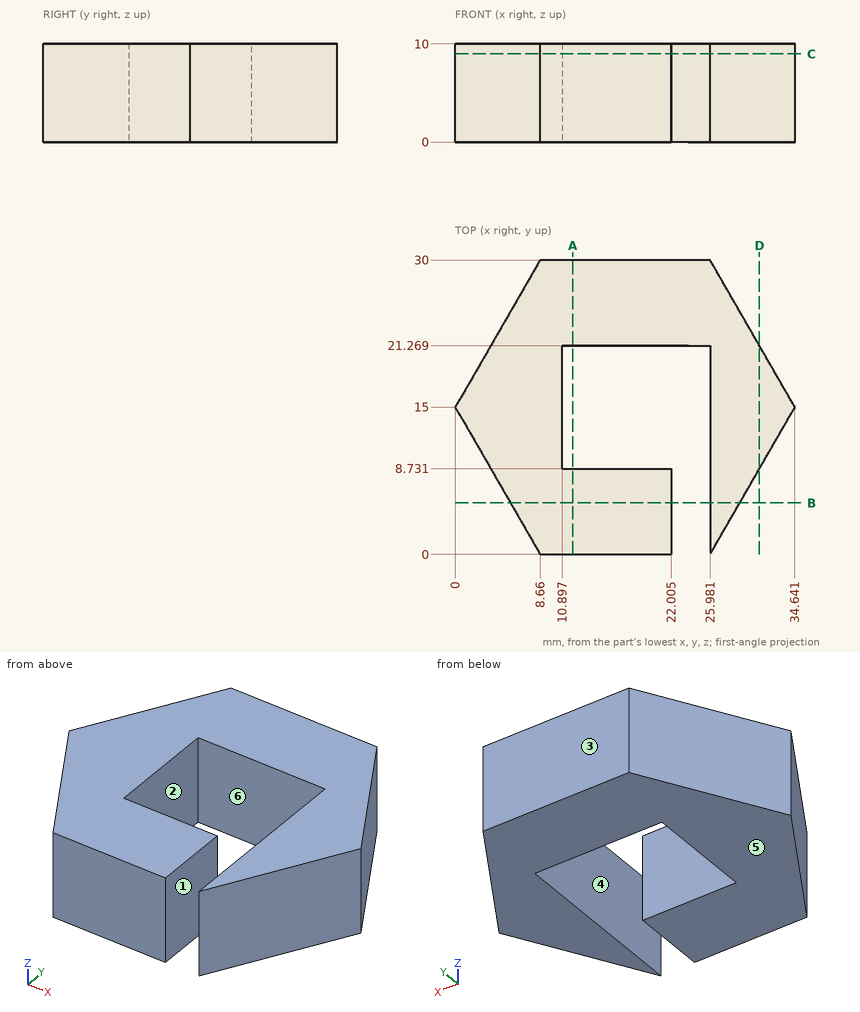
Verification items for this drawing (mm, ordinates from the low corner). A direction names the side the tool comes from. Coordinates: 2 decimals unless noted, no trailing zeros. Order: outer loops, then holes, each group sorted by start corner. A loop starts at its lowest first (then second) coordinate and runs counter-clockwise, first axis right, second up. Notation, with made-up numbers: (35.5, -31.5) - (50.5, -31.5) arc R13 ccw to (50.5, -7.5) - close; hole circle Ø7 at (61, -1). An arc over 180 degrees is marked (long way). Answer in a Markdown table with one row per item. Add a question column.
1. Section check C-C (z = 9). Enter the section's corners in (x, y) (1 decimal).
2. Material ranges on L1, parallel to Y at x = 17.5, z = 6.75; L2, parallel to X at y = 19.25, z = 5 (1 decimal); L3, parallel to X at y = 9.5, z = 2.25 (1 decimal), recorded low to high. Write a range as [from, to].
3. Draft check along Y on the marked faces 1, 2 and 3. Enter one of: +Y half, -Y half, draft (parallel to the pull), parting line (faces both ways), or undercut.
4. Section check B-B (y = 5.25). Enter the section's corners in (x, z) (1 decimal), plus the area to 3 significant figures.
5. Access from +Z, -Z, +X, -X, +Y, -Y to the whole of each face (thin tool, end or side, straight path). Record for the marked faces 4, 5 and 6.
6. Section check D-D (x = 31). Enter the section's corners in (y, z), plus the area to 3 significant figures.
7. Section check A-A (x = 12). Enter the section's corners in (y, z), plus the area to 3 significant figures.
8. Gauge pin test, flat ends, axial feed: pin 1 Ø4 at (y, z) = (5.5, 6) entering from -X; pin 2 Ø3 at (y, z) = (13, 7) entering from +X; pin 3 Ø2 at (y, z) = (3.5, 3) entering from +X. Record the tip position at first contact, or that the pin passes through.
Data:
| question | item | result |
|---|---|---|
| 1 | outline | (0, 15) - (8.7, 0) - (22, 0) - (22, 8.7) - (10.9, 8.7) - (10.9, 21.3) - (26, 21.3) - (26, 0) - (34.6, 15) - (26, 30) - (8.7, 30) - close |
| 2 | L1 | y = [0, 8.73], [21.27, 30] |
| 2 | L2 | x = [2.5, 10.9], [26, 32.2] |
| 2 | L3 | x = [3.2, 10.9], [26, 31.5] |
| 3 | face 1 | draft |
| 3 | face 2 | undercut |
| 3 | face 3 | +Y half |
| 4 | outline | (5.6, 0) - (22, 0) - (22, 10) - (5.6, 10) - close; (26, 0) - (29, 0) - (29, 10) - (26, 10) - close |
| 4 | area | 194 mm² |
| 5 | face 4 | +Z, -Z, -Y |
| 5 | face 5 | -Z, +X, -X, +Y, -Y |
| 5 | face 6 | +Z, -Z |
| 6 | outline | (8.69, 0) - (21.31, 0) - (21.31, 10) - (8.69, 10) - close |
| 6 | area | 126 mm² |
| 7 | outline | (0, 0) - (8.73, 0) - (8.73, 10) - (0, 10) - close; (21.27, 0) - (30, 0) - (30, 10) - (21.27, 10) - close |
| 7 | area | 175 mm² |
| 8 | pin 1 | stops at x = 4.33 |
| 8 | pin 2 | stops at x = 34.35 |
| 8 | pin 3 | stops at x = 28.58 |
